from build123d import *

# Parameters (mm, degrees)
BOSS_EXTRUDE1_DEPTH = 29
CHAMFER1_SIZE       = 0.8


with BuildPart() as part:
    # Sketch1 → Boss-Extrude1 (new body)
    with BuildSketch(Plane(origin=(0, 0, 0), x_dir=(1, 0, 0), z_dir=(0, 1, 0))):
        with BuildLine():
            Line((-0.5, -5), (-0.5, -9.486832981))
            ThreePointArc((-0.5, -9.486832981), (0, 9.5), (0.5, -9.486832981))
            Line((0.5, -9.486832981), (0.5, -5))
            Line((0.5, -5), (0.5, -4.974937186))
            ThreePointArc((0.5, -4.974937186), (0, 5), (-0.5, -4.974937186))
            Line((-0.5, -4.974937186), (-0.5, -5))
        make_face()
    extrude(amount=BOSS_EXTRUDE1_DEPTH)

    # Chamfer1
    chamfer1_edges = [part.edges().sort_by_distance(p)[0] for p in [
        (0, 29, -9.5),
        (0, 0, -9.5),
    ]]
    chamfer(chamfer1_edges, length=CHAMFER1_SIZE)


solid = part.part
CAD build for the part. Positions are in the model's coordinates, mm. A direction names the side the tool comes from. Give positions to 0.01 mm unless a question says otherwise; leave off trailing zeros. Write each loop counter-clockwise with the first axis right and the second up, starting at its lowest first coordinate (ties: lowest second). Pieces come first, ordered by that corner, then holes. Notation, with made-up numbers: M 71,52 L 97,52 A36 ccw 97,88 Z; hole C -12.75,-23.75 d1. An arc over 180 degrees is marked long. Put each result on its own line as item: value. Start each with the question number.
(1) Flat gauge pins, fed straight in: pin 1 Ø1.5 at (y, z) = (23.5, -4.5) entering from +X; pin 2 Ø8 at (x, z) = (0, 0) entering from +Y; pin 3 Ø1.5 at (x, y) = (4.5, 15.5) entering from -Z; pin 4 Ø3.5 at (y, z) = (9, 6) entering from +X. Where does each tip first touch, or does it go through?
(2) Which spindle directions (+Z, -Z, +X, -X, +Y, -Y) get a long thin tool onto all of the face, cutting with end or side? Do faces 4 (the face through (0.5, 14, 7)), 5 (the face through (-4, 29, 4)). Say none if no direction does.
(3) Probe L1, parallel to X at y = 16, z = 0; L2, parallel to X at y = 19.5, z = -3.5; L3, parallel to Z at x = -2.75, y = 10.75. List the from-to ranges inside material, lowest first.
(4) Band-saw the part on A-A, the plane z = 0. Write the cut outline in (x, y), and give its area (3 significant figures).
(5) Mould opens along X. For faces 1 (the face through (-0.5, 14, 7)), 2 (the face through (-0.38, 0.13, -8.82)), 3 (the face through (-4, 0, 4)) say: +X half, -X half, draft (parallel to the pull), parting line (faces both ways), or undercut.
(6) Band-saw the part on B-B, the plane x = 0. Write the cut outline in (y, z).
(7) Band-saw the part on C-C, the plane y = 22.5. Write the cut outline in (x, z), and give its area (3 significant figures).
Response values:
1. pin 1: stops at x = 8.73
1. pin 2: passes through
1. pin 3: stops at z = -8.73
1. pin 4: stops at x = 8.5
2. face 4: +Z, +Y, -Y
2. face 5: +Z, -Z, +X, -X, +Y
3. L1: x = -9.5 to -5, 5 to 9.5
3. L2: x = -8.83 to -3.57, 3.57 to 8.83
3. L3: z = -9.09 to -4.18, 4.18 to 9.09
4. outline: M -9.5,0.8 L -8.7,0 L -5,0 L -5,29 L -8.7,29 L -9.5,28.2 Z; M 5,0 L 8.7,0 L 9.5,0.8 L 9.5,28.2 L 8.7,29 L 5,29 Z
4. area: 260 mm2
5. face 1: undercut
5. face 2: parting line
5. face 3: draft
6. outline: M 0,-8.7 L 0.8,-9.5 L 28.2,-9.5 L 29,-8.7 L 29,-5 L 0,-5 Z
7. outline: M -0.5,4.97 L -0.5,9.49 A9.5 ccw long 0.5,9.49 L 0.5,4.97 A5 cw long Z
7. area: 200 mm2
